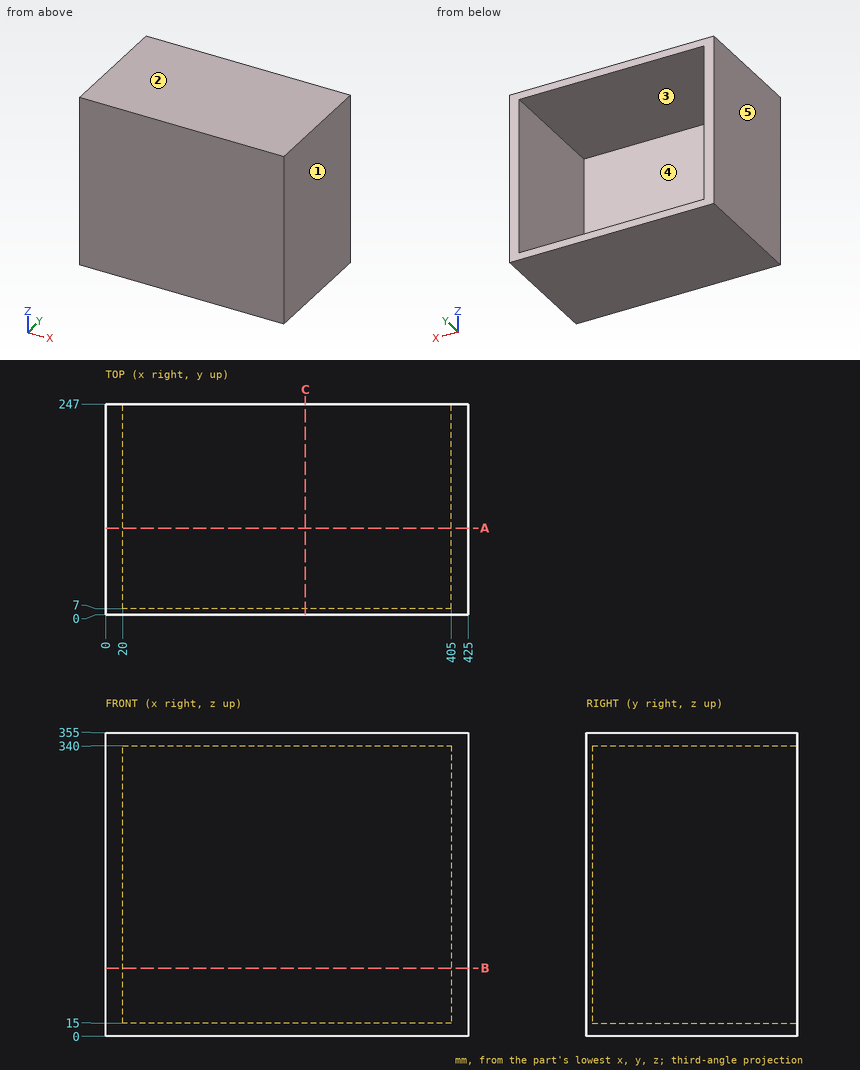
Answer from the drawing. Dimensions are ordinates in mm from the lowest x, y and z of the part. A direction names the side the tool comes from. Coordinates: 2 decimals unless noted, no trailing zeros. Loops run counter-clockwise (first coordinate to the right, second up) from the corner with the lowest first, then second, coordinate; pieces in that order, holes last. Notation, with made-up numbers: (81, -4) - (116, -4) arc R21 cw to (116, 14) - close; hole circle Ø5 at (43, 52.5). An arc over 180 degrees is marked (long way). Use a Markdown table: item, result.
Item 1: Given pin 1 Ø2 at (x, z) = (51, 271.5) entering from +Y, flat-ended and moving along its own axis, determine where the tip first touches the part or whether it passes through.
Evaluation:
| item | result |
|---|---|
| pin 1 | stops at y = 7 |
Item 2: Find section A-A, the plane y = 101.5. Determine the outline of the cut face in (x, z).
Evaluation:
| item | result |
|---|---|
| outline | (0, 0) - (425, 0) - (425, 355) - (0, 355) - close; hole (20, 15) - (405, 15) - (405, 340) - (20, 340) - close |
Item 3: Find section B-B, the plane z = 79.5. Determine the outline of the cut face in (x, y), and give its area (3 significant figures).
Evaluation:
| item | result |
|---|---|
| outline | (0, 0) - (425, 0) - (425, 247) - (405, 247) - (405, 7) - (20, 7) - (20, 247) - (0, 247) - close |
| area | 12,600 mm2 |
Item 4: Consider probe 1 along Z at (x, y) = (36.5, 68.5); probe 2 along X at (y, z) = (94.5, 39); probe 3 along Y at (x, z) = (104.5, 61). Determine where each line is inside the solid, lowest interval first. Write a range as from..to.
Evaluation:
| item | result |
|---|---|
| probe 1 | z = 0..15, 340..355 |
| probe 2 | x = 0..20, 405..425 |
| probe 3 | y = 0..7 |
Item 5: For the marked faces 4 and 5, determine the directions among +Z, -Z, +X, -X, +Y, -Y from which every point of the face is accessible in a straight line to the end or side of a thin tool.
Evaluation:
| item | result |
|---|---|
| face 4 | +Y |
| face 5 | +Z, -Z, -X, +Y, -Y |
Item 6: Find section C-C, the plane x = 234. Determine the outline of the cut face in (y, z), and give its area (4 significant figures).
Evaluation:
| item | result |
|---|---|
| outline | (0, 0) - (247, 0) - (247, 15) - (7, 15) - (7, 340) - (247, 340) - (247, 355) - (0, 355) - close |
| area | 9,685 mm2 |
Item 7: The mould has two halves that part along X. Classify the marked faces 1, 2 and 3: +X half, -X half, draft (parallel to the pull), parting line (faces both ways), or undercut.
Evaluation:
| item | result |
|---|---|
| face 1 | +X half |
| face 2 | draft |
| face 3 | undercut |
